from build123d import *

# Parameters (mm, degrees)
F0_W     = 63.5
F0_H     = 12.7
F1_DEPTH = 63.5
F2_W     = 13.266523
F2_H     = 22.422786
F3_DEPTH = 63.5
F4_W     = 12.7
F4_H     = 12.7
F5_DEPTH = 25.4
F6_W     = 12.7
F6_H     = 12.7
F7_DEPTH = 25.4


with BuildPart() as f1:
    # F0 (on Front) → F1 (new body)
    with BuildSketch(Plane.XZ):
        with Locations((-6.000457, 6.35)):
            Rectangle(F0_W, F0_H)
    extrude(amount=F1_DEPTH)

    # F2 (on Front) → F3 (join)
    with BuildSketch(Plane.XZ):
        with Locations((-31.117195, 23.911393)):
            Rectangle(F2_W, F2_H)
    extrude(amount=F3_DEPTH)

    # F4 (on face) → F5 (join)
    with BuildSketch(Plane.YZ.offset(-24.483934)):
        with Locations((-57.15, 19.05)):
            Rectangle(F4_W, F4_H)
    extrude(amount=F5_DEPTH)

    # F6 (on face) → F7 (join)
    with BuildSketch(Plane.YZ.offset(-24.483934)):
        with Locations((-6.35, 19.05)):
            Rectangle(F6_W, F6_H)
    extrude(amount=F7_DEPTH)


solid = f1.part
The listing builds one solid part. Answer for the finished solid, in the listing's coordinates (mm). A direction names the side the tool comes from. Round coordinates to 2 decimals unless told otherwise and drop trailing zeros. Order: outer loops, then holes, each group sorted by start corner. A loop starts at its lowest first (then second) coordinate and runs counter-clockwise, first axis right, second up. Notation, with made-up numbers: M -28.5,22.5 L -18.5,22.5 A22 cw -18.5,49.5 Z; hole C 58.5,-24 d4. An arc over 180 degrees is marked long. Answer in a Markdown table with one row per item. Add a question column.
1) The part is cut by section D-D on y = -39. Determine the outline of the cut face in (x, z).
2) The part is cut by section C-C on x = 9.5. Determine the outline of the cut face in (y, z), plus the area to 3 significant figures.
3) Determine the mould class of faces 1 (the face through (-14, -63.5, 14)), 2 (the face through (-14, 0, 14)), 3 (the face through (0.916, -6, 19)), 4 (the face through (-12, -50.8, 19)) for opening direction Y: pulls with the +Y half, pulls with the -Y half, needs draft (parallel to the pull), parting line crosses it, or undercut.
4) The part is cut by section A-A on z = 20.5. Determine the outline of the cut face in (x, y), plus the area to 3 significant figures.
5) The part is cut by section B-B on y = -54. Determine the outline of the cut face in (x, z), plus the area to 3 significant figures.
6) Consider line 1 along Y through (x, z) = (-16.5, 14); line 2 along X through (y, z) = (-19.5, 14); line 3 along Z through (x, y) = (8, -7.5). Determine where each line is inside the solid, lowest interval first. Write a range as from..to.
7) Flat-ended cylindrical pins translate along their axes: pin 1 Ø6.5 at (y, z) = (-4, 20.5) entering from +X; pin 2 Ø2 at (x, z) = (-3, 10.5) entering from +Y; pin 3 Ø14 at (x, y) = (-11.5, -9) entering from +Z; pin 4 Ø15 at (x, y) = (-9, -39.5) entering from +Z. Find the tip coordinate at first contact, or state that the pin passes through.
8) Which of the six approach directions +Z, -Z, +X, -X, +Y, -Y give full straight-line access (tool end or side, diameter ignored) to faces 5 (the face through (-37.75, -31, 6)), 6 (the face through (-12, -57, 25.4)), 7 (the face through (-12, -12.7, 19))?
Findings below:
| question | item | result |
|---|---|---|
| 1 | outline | M -37.75,0 L 25.75,0 L 25.75,12.7 L -24.48,12.7 L -24.48,35.12 L -37.75,35.12 Z |
| 2 | outline | M -63.5,0 L 0,0 L 0,12.7 L -63.5,12.7 Z |
| 2 | area | 806 mm² |
| 3 | face 1 | pulls with the -Y half |
| 3 | face 2 | pulls with the +Y half |
| 3 | face 3 | needs draft |
| 3 | face 4 | undercut |
| 4 | outline | M -37.75,-63.5 L 0.92,-63.5 L 0.92,-50.8 L -24.48,-50.8 L -24.48,-12.7 L 0.92,-12.7 L 0.92,0 L -37.75,0 Z |
| 4 | area | 1,490 mm² |
| 5 | outline | M -37.75,0 L 25.75,0 L 25.75,12.7 L 0.92,12.7 L 0.92,25.4 L -24.48,25.4 L -24.48,35.12 L -37.75,35.12 Z |
| 5 | area | 1,430 mm² |
| 6 | line 1 | y = -63.5..-50.8, -12.7..0 |
| 6 | line 2 | x = -37.75..-24.48 |
| 6 | line 3 | z = 0..12.7 |
| 7 | pin 1 | stops at x = 0.92 |
| 7 | pin 2 | stops at y = 0 |
| 7 | pin 3 | stops at z = 25.4 |
| 7 | pin 4 | stops at z = 12.7 |
| 8 | face 5 | +Z, -Z, -X, +Y, -Y |
| 8 | face 6 | +Z, +X, +Y, -Y |
| 8 | face 7 | +Z, +X |
